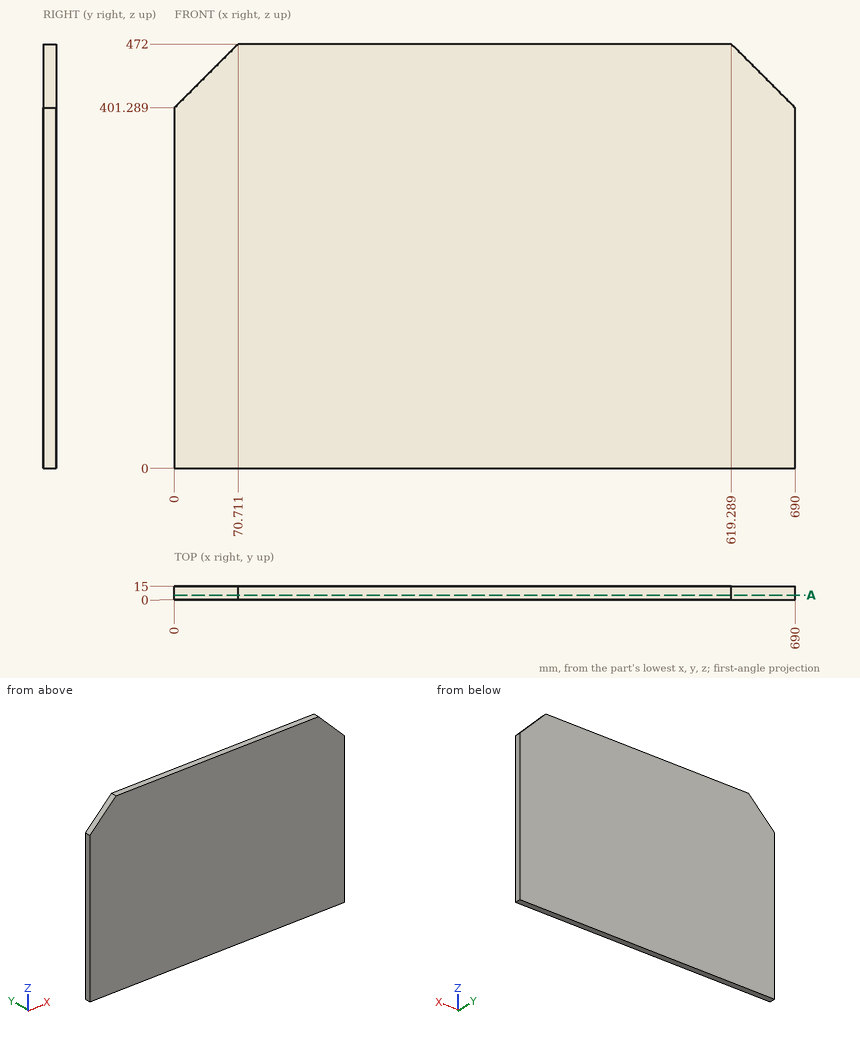
Answer from the drawing. Dimensions are ordinates in mm from the lowest x, y and z of the part. Give positions to 0.01 mm unless a question says otherwise; leave off trailing zeros. Order: outer loops, then holes, each group sorted by start corner. A loop starts at its lowest first (then second) coordinate and runs counter-clockwise, first axis right, second up.
Item 1: Find the intervals of material crossed by probe 1 along Z at (x, y) = (45, 9); probe 2 along X at (y, z) = (12, 419), in increasing order.
From the geometry:
probe 1: z = 0 to 446.29
probe 2: x = 17.71 to 672.29
Item 2: The part is cut by section A-A, the plane y = 5.25. Give the vertices of the cut face in (x, z).
From the geometry:
outline: (0, 0) - (690, 0) - (690, 401.29) - (619.29, 472) - (70.71, 472) - (0, 401.29) - close
Item 3: Given pin 1 Ø1.5 at (x, z) = (171.5, 218.5) entering from -Y; pin 2 Ø6 at (y, z) = (9, 413.5) entering from -X, each flat-ended and moving along its own axis, determine where each tip first touches the part or whether it passes through.
From the geometry:
pin 1: stops at y = 0
pin 2: stops at x = 9.21
